Could you check a few things on this model? Use its own coordinates, in mm. A direction names the side the tool comes from. Round coordinates to 2 decimals unless told otherwise and drop trailing zeros. Order: outer loops, then holes, each group sorted by start corner. A loop starts at its lowest first (then second) coordinate and runs counter-clockwise, first axis right, second up. Notation, with made-up numbers: (79, 19) - (113, 19) arc R21 ccw to (113, 42) - close; hole circle Ø8 at (34, 23.5). An arc over 180 degrees is marked (long way). Use one line per item in the form item = value.
from build123d import *

# Parameters (mm, degrees)
FUNNEL_LEFT_SIDE_DEPTH = 155
FILLET1_R              = 10


with BuildPart() as part:
    # Sketch1 → Funnel - Left Side (new body)
    with BuildSketch(Plane.XY):
        with BuildLine():
            Line((-5, 1.037386495), (-5, 70.037386495))
            Line((-5, 70.037386495), (-46.974030913, 120.060088631))
            Line((-46.974030913, 120.060088631), (-41.974030913, 120.060088631))
            Line((-41.974030913, 120.060088631), (0, 70.037386495))
            Line((0, 70.037386495), (0, 0))
            ThreePointArc((0, 0), (-2.495861145, 0.538641718), (-5, 1.037386495))
        make_face()
    extrude(amount=FUNNEL_LEFT_SIDE_DEPTH)

    # Fillet1
    fillet1_edges = [part.edges().sort_by_distance(p)[0] for p in [
        (-5, 70.037386495, 77.5),
        (0, 70.037386495, 77.5),
    ]]
    fillet(fillet1_edges, radius=FILLET1_R)


solid = part.part
Item 1: For faces 1 (the face through (-45, 120.06, 76)), 2 (the face through (-5, 33, 76)), which set-ups out of +Z, -Z, +X, -X, +Y, -Y let a thin tool reach every point of the face, with its end or its side?
Found:
face_1 = +Z, -Z, +X, -X, +Y
face_2 = +Z, -Z, -X, -Y
Item 2: Will these pins go through, and if not, where does the flat tip stop? P1, Ø1, axis at y = 104, z = 80.5, coming from the -X side; P2, Ø2, axis at x = -40, z = 121, coming from the -Y side; P3, Ø1, axis at y = 48, z = 60, coming from the -X side.
Found:
P1 = -33.92
P2 = 110.56
P3 = -5
Item 3: Imagine slicing it at A-A on z = 142. Please give me the cut outline in (x, y).
Found:
outline = (-46.97, 120.06) - (-7.34, 72.83) arc R10 cw to (-5, 66.4) - (-5, 1.04) arc R160 cw to (0, 0) - (0, 66.4) arc R10 ccw to (-2.34, 72.83) - (-41.97, 120.06) - close
Item 4: Imagine slicing it at B-B on x = -14. Please give me the cut outline in (y, z), plus the area to 3 significant figures.
Found:
outline = (80.76, 0) - (86.72, 0) - (86.72, 155) - (80.76, 155) - close
area = 924 mm2
Item 5: Imagine slicing it at C-C on y = 71. Please give me the cut outline in (x, z).
Found:
outline = (-6.12, 0) - (-1.12, 0) - (-1.12, 155) - (-6.12, 155) - close
Item 6: I need wall thicknesses on L1, parallel to X at y = 15.5, z = 51; L2, parallel to Y at x = -16, z = 121.5; L3, parallel to Y at x = -22, z = 95.5. Which ranges of each line are inside material? Lowest first, please.
Found:
L1 = -5 to 0
L2 = 83.15 to 89.11
L3 = 90.3 to 96.26
